from build123d import *

# Parameters (mm, degrees)
F0_W     = 36.725904
F0_H     = 71.635686
F1_DEPTH = 29.21


with BuildPart() as f1:
    # F0 (on Right) → F1 (new body, symmetric)
    with BuildSketch(Plane.YZ):
        Rectangle(F0_W, F0_H)
        Polygon((-18.362952, 35.817843), (18.362952, 35.817843), (5.246557, 45.302007), (5.246557, 51.557515), (0, 51.557515), (-5.246557, 51.557515), (-5.246557, 45.302007), align=None)
    extrude(amount=F1_DEPTH, both=True)


solid = f1.part
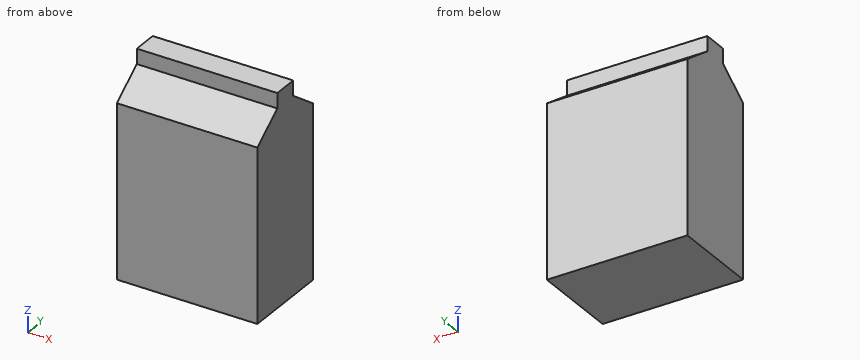
Input: part model. Units: mm. Frame: model coordinates. Coordinates: 2 decimals unless noted, no trailing zeros. Order: outer loops, then holes, each group sorted by start corner. A loop starts at its lowest first (then second) coordinate and runs counter-clockwise, first axis right, second up.
1. Contact query for flat-ended pins moving along their axis: P1, Ø5, axis at x = -22, z = 40, coming from the -Y side; P2, Ø5, axis at x = -8, z = 47.5, coming from the +Y side; P3, Ø3, axis at x = -8.5, z = 47.5, coming from the -Y side. Output: stop coordinate, or through.
Checked values:
P1: stops at y = -16.04
P2: stops at y = 5.66
P3: stops at y = -5.25
2. Ray query, line 1 along Z through (x, y) = (25, 6); line 2 along Z through (x, y) = (7.5, 7); line 3 along Y through (x, z) = (-3, 39). Return the intervals inside material, ascending.
Checked values:
line 1: z = -35.82 to 44.76
line 2: z = -35.82 to 44.03
line 3: y = -13.96 to 13.96
3. Cut plane B-B, the plane y = 10. Return loops of the section in (x, z).
Checked values:
outline: (-29.21, -35.82) - (29.21, -35.82) - (29.21, 41.86) - (-29.21, 41.86) - close
4. Cut plane A-A, the plane x = -17. Return loops of the section in (y, z).
Checked values:
outline: (-18.36, -35.82) - (18.36, -35.82) - (18.36, 35.82) - (5.25, 45.3) - (5.25, 51.56) - (-5.25, 51.56) - (-5.25, 45.3) - (-18.36, 35.82) - close
